Part model, mm, in its own coordinate system. A direction names the side the tool comes from. Round coordinates to 2 decimals unless told otherwise and drop trailing zeros. Write each loop counter-clockwise with the first axis right and the second up, starting at its lowest first coordinate (ties: lowest second). Pieces come first, ordered by that corner, then holes. Notation, with made-up numbers: M 29,-30.5 L 40,-30.5 A21 cw 40,-15.5 Z; hole C 82.5,67.25 d1. An arc over 180 degrees is marked long. Answer as a JSON object with one key per item and string values. Group by question number.
1. Drop flat-ended pins along their axis: pin 1 (4 mm diameter, centred on x = 0, y = 18, fed in from +Z); pin 2 (3 mm diameter, centred on y = -4, z = 2.5, fed in from +X); pin 3 (1 mm diameter, centred on x = 14.5, z = 14, fed in from -Y). Give the stop position or say it passes through.
2. Which spindle directions (+Z, -Z, +X, -X, +Y, -Y) get a long thin tool onto all of the face, cutting with end or side? Do faces 4 (the face through (2.385, -17.249, 17.605)), 5 (the face through (0, -1, 21)), 6 (the face through (0, 0, 25)), 7 (the face through (0, 14, 9)). Say none if no direction does.
3. Band-saw the part on D-D, the plane y = 9. Write the cut outline in (x, z), plus the area to 3 significant figures.
4. Drill centre lines: line 1 (Y direction, x = 13.5, z = 17); line 2 (X direction, y = 10.5, z = 15.75); line 3 (Y direction, x = 1, z = 20.5). Where is each one in solid material? Low to high. Write a range as from..to.
5. Band-saw the part on B-B, the plane z = 17.25. Write the cut outline in (x, y).
6. Band-saw the part on A-A, the plane x = 0. Write the cut outline in (y, z), plus the area to 3 significant figures.
7. Two-plate mould, pull along Y, no slides. Class faces 1 (the face through (-2.994, 22.804, 12.325)), 2 (the face through (-17.572, 7.479, 17.605)), 3 (the face through (0, 5, 0)): +Y half, -Y half, draft (parallel to the pull), parting line (faces both ways), or undercut.
8. Band-saw the part on C-C, the plane y = 18. Write the cut outline in (x, z).
from build123d import *

# Parameters (mm, degrees)
F0_R     = 23
F4_DEPTH = 25
F6_R     = 2.5
F1_DEPTH = 15
F2_DEPTH = 4
F8_R     = 1.5
F3_DEPTH = 35


# Not quite as in the source:
# - a feature names something its author has since deleted; it is built from what else it names


with BuildPart() as f4:
    # F0 (on Top) → F4 (new body)
    with BuildSketch(Plane.XY):
        Circle(F0_R)
        with BuildLine():
            ThreePointArc((4.85, 3.616628264), (5.7421685799, 1.9052558883), (6.05, 0))
            ThreePointArc((6.05, 0), (5.7421685799, -1.9052558883), (4.85, -3.616628264))
            Line((4.85, -3.616628264), (4.85, -4.85))
            Line((4.85, -4.85), (3.616628264, -4.85))
            ThreePointArc((3.616628264, -4.85), (0, -6.05), (-3.616628264, -4.85))
            Line((-3.616628264, -4.85), (-4.85, -4.85))
            Line((-4.85, -4.85), (-4.85, -3.616628264))
            ThreePointArc((-4.85, -3.616628264), (-6.05, 0), (-4.85, 3.616628264))
            Line((-4.85, 3.616628264), (-4.85, 4.85))
            Line((-4.85, 4.85), (-3.616628264, 4.85))
            ThreePointArc((-3.616628264, 4.85), (0, 6.05), (3.616628264, 4.85))
            Line((3.616628264, 4.85), (4.85, 4.85))
            Line((4.85, 4.85), (4.85, 3.616628264))
        make_face(mode=Mode.SUBTRACT)
        with BuildLine():
            ThreePointArc((3.616628264, 4.85), (4.2779960262, 4.2779960262), (4.85, 3.616628264))
            Line((4.85, 3.616628264), (4.85, 4.85))
            Line((4.85, 4.85), (3.616628264, 4.85))
        make_face()
        with BuildLine():
            Line((-3.616628264, 4.85), (3.616628264, 4.85))
            ThreePointArc((3.616628264, 4.85), (0, 6.05), (-3.616628264, 4.85))
        make_face()
        with BuildLine():
            ThreePointArc((-4.85, 3.616628264), (-4.2779960262, 4.2779960262), (-3.616628264, 4.85))
            Line((-3.616628264, 4.85), (-4.85, 4.85))
            Line((-4.85, 4.85), (-4.85, 3.616628264))
        make_face()
        with BuildLine():
            Line((-4.85, -4.85), (-3.616628264, -4.85))
            ThreePointArc((-3.616628264, -4.85), (-4.2779960262, -4.2779960262), (-4.85, -3.616628264))
            Line((-4.85, -3.616628264), (-4.85, -4.85))
        make_face()
        with BuildLine():
            Line((4.85, -4.85), (4.85, -3.616628264))
            ThreePointArc((4.85, -3.616628264), (4.2779960262, -4.2779960262), (3.616628264, -4.85))
            Line((3.616628264, -4.85), (4.85, -4.85))
        make_face()
    extrude(amount=F4_DEPTH)

    # F6 (on face) → F1 (cut)
    with BuildSketch(Plane.XY.offset(25)):
        with Locations((15.5884572681, 9)):
            Circle(F6_R)
        with Locations((0, 18)):
            Circle(F6_R)
        with Locations((-15.5884572681, 9)):
            Circle(F6_R)
        with Locations((15.5884572681, -9)):
            Circle(F6_R)
        with Locations((0, -18)):
            Circle(F6_R)
        with Locations((-15.5884572681, -9)):
            Circle(F6_R)
    extrude(amount=-F1_DEPTH, mode=Mode.SUBTRACT)

    # F7 (on face) → F2 (join)
    with BuildSketch(Plane.XY.offset(25)):
        with BuildLine():
            Line((3.616628264, 4.85), (-3.616628264, 4.85))
            ThreePointArc((-3.616628264, 4.85), (0, -6.05), (3.616628264, 4.85))
        make_face()
    extrude(amount=-F2_DEPTH)

    # F8 (on face) → F3 (cut)
    with BuildSketch(Plane.XZ.offset(-4.85)):
        with Locations((0, 10.5)):
            Circle(F8_R)
    extrude(amount=-F3_DEPTH, mode=Mode.SUBTRACT)


solid = f4.part
Worked answers:
{
 "1": {"pin 1": "stops at z = 10", "pin 2": "stops at x = 22.86", "pin 3": "stops at y = -18.25"},
 "2": {"face 4": "+Z", "face 5": "-Z", "face 6": "+Z, +X, -X, +Y, -Y", "face 7": "+Y"},
 "3": {"outline": "M -21.17,0 L 21.17,0 L 21.17,25 L 18.09,25 L 18.09,10 L 13.09,10 L 13.09,25 L -13.09,25 L -13.09,10 L -18.09,10 L -18.09,25 L -21.17,25 Z; hole C 0,10.5 d3", "area": "901 mm^2"},
 "4": {"line 1": "y = -18.62..-10.37, -7.63..7.63, 10.37..18.62", "line 2": "x = -20.46..-17.59, -13.59..13.59, 17.59..20.46", "line 3": "y = -22.98..-20.29, -15.71..-5.97, 4.85..15.71, 20.29..22.98"},
 "5": {"outline": "C 0,0 d46; hole C -15.59,-9 d5; hole C -15.59,9 d5; hole M -3.62,4.85 A6.05 ccw long 3.62,4.85 Z; hole C 0,-18 d5; hole C 0,18 d5; hole C 15.59,-9 d5; hole C 15.59,9 d5"},
 "6": {"outline": "M -23,0 L -6.05,0 L -6.05,21 L 4.85,21 L 4.85,12 L 15.5,12 L 15.5,25 L -15.5,25 L -15.5,10 L -20.5,10 L -20.5,25 L -23,25 Z; M 4.85,0 L 23,0 L 23,9 L 4.85,9 Z; M 20.5,12 L 23,12 L 23,25 L 20.5,25 Z", "area": "727 mm^2"},
 "7": {"face 1": "parting line", "face 2": "undercut", "face 3": "draft"},
 "8": {"outline": "M -14.32,0 L 14.32,0 L 14.32,25 L 2.5,25 L 2.5,10 L 1.41,10 A1.5 cw -1.41,10 L -2.5,10 L -2.5,25 L -14.32,25 Z"}
}
